```python
from build123d import *

# Parameters (mm, degrees)
F0_W      = 38.1
F0_H      = 38.1
F1_DEPTH  = 38.1
F6_DEPTH  = 38.1
F8_DEPTH  = 38.1
F9_W      = 25.4
F9_H      = 7.62
F10_DEPTH = 38.1


with BuildPart() as f1:
    # F0 (on Front) → F1 (new body)
    with BuildSketch(Plane.XZ):
        with Locations((-19.05, 19.05)):
            Rectangle(F0_W, F0_H)
    extrude(amount=F1_DEPTH)

    # F5 (on offset) → F6 (cut)
    with BuildSketch(Plane.YZ.offset(-38.1)):
        Polygon((-11.43, 13.500985), (-6.35, 38.1), (-31.75, 38.1), (-26.67, 13.624078), (-21.59, 28.575), (-16.51, 28.575), align=None)
        Polygon((-25.4, 0), (-12.7, 0), (-19.05, 15.875), align=None)
        Polygon((-6.35, 0), (0, 0), (0, 38.1), align=None)
        Polygon((-31.75, 0), (-38.1, 38.1), (-38.1, 0), align=None)
    extrude(amount=F6_DEPTH, mode=Mode.SUBTRACT)

    # F7 (on offset) → F8 (cut)
    with BuildSketch(Plane.XZ.offset(38.1)):
        Polygon((-31.75, 0), (-6.35, 0), (-11.43, 19.455044), (-16.51, 9.525), (-21.59, 9.525), (-26.67, 19.085767), align=None)
        Polygon((-6.35, 38.1), (0, 0), (0, 38.1), align=None)
        Polygon((-19.05, 22.225), (-12.7, 38.1), (-25.4, 38.1), align=None)
        Polygon((-38.1, 38.1), (-38.1, 0), (-31.75, 38.1), align=None)
    extrude(amount=-F8_DEPTH, mode=Mode.SUBTRACT)

    # F9 (on offset) → F10 (cut)
    with BuildSketch(Plane.XY.offset(38.1)):
        with Locations((-12.7, -11.43)):
            Rectangle(F9_W, F9_H)
        with Locations((-25.4, -26.67)):
            Rectangle(F9_W, F9_H)
    extrude(amount=-F10_DEPTH, mode=Mode.SUBTRACT)


solid = f1.part
```
For this review, take the finished solid that the model builds, in its own axes (mm). A direction names the side the tool comes from. Round coordinates to 2 decimals unless told otherwise and drop trailing zeros. Write each loop counter-clockwise with the first axis right and the second up, starting at its lowest first coordinate (ties: lowest second). Pieces come first, ordered by that corner, then holes. Notation, with made-up numbers: (16, 5) - (55, 5) arc R6 cw to (55, 9) - close; hole circle Ø10 at (43, 80.25). An arc over 180 degrees is marked (long way). Answer as CSV lines item,"result". Start each with the question number.
(1) Add section D-D, the plane z = 12. State how many separate pieces and enclosed holes the cut face has, plus the area to 3 significant figures.
(2) For line 1 (Y direction, x = -26.5, z = 23.5); line 2 (Y direction, x = -11.5, z = 21); line 3 (X direction, y = -22.5, z = 10.5), list the stretches that pass through material, from the lowest coordinate up.
(3) Add section A-A, the plane x = -3.5. State the section outline as (y, z) points (3 decimals).
(4) Mouldability with a two-part tool opening along Y and no side actions: class faces 6 (the flat face through (-22.27, -33.5, 30.27)), 7 (the flat face through (-19.32, -34.88, 18.78)), 8 (the flat face through (-26, -30.48, 20)) as +Y half, -Y half, draft (parallel to the pull), parting line (faces both ways), or undercut.
(5) Add section B-B, the plane z = 30.5. State the section outline as (x, y) points, plus the area to 3 significant figures.
(6) Add section C-C, the plane y = -9.5. State the section outline as (x, z) points.
(7) For pin 1 (2 mm diameter, centred on x = -32, z = 10, fed in from -Y); pin 2 (2.5 mm diameter, centred on x = -13, y = -18.5, fed in from +Z) (3 decimals); pin 3 (8 mm diameter, centred on x = -28.5, y = -34, fed in from -Z); pin 4 (2 mm diameter, centred on y = -23.5, z = 19.5, fed in from -X), all flat-tipped, find the tip position at first contact; note any pin that passes through.
(8) Machinability: for faces 1 (the flat face through (-4, -5, 24)), 2 (the flat face through (-13.934, -5.897, 14.56)), 3 (the flat face through (-27.93, -31.124, 35.083)), 4 (the flat face through (-15.9, -33.5, 30.1)), 5 (the flat face through (-19.195, -18.044, 13.361)), which of the approach directions +Z, -Z, +X, -X, +Y, -Y give a long, thin tool a straight path to every point of the face, cutting with its end or side? Answer none if there is none.
From the geometry:
1,separate pieces,"10"
1,enclosed holes,"0"
1,area,"365 mm²"
2,line 1,"y = -35.67 to -30.48, -22.86 to -14.8, -9.37 to -2.43"
2,line 2,"y = -35.25 to -28.2, -24.16 to -15.24, -7.62 to -2.85"
2,line 3,"x = -36.35 to -28.96, -22.11 to -16.01, -9.09 to -1.75"
3,outline,"(-35.25, 21) - (-31.75, 0) - (-25.4, 0) - (-19.05, 15.875) - (-15.24, 6.35) - (-15.24, 21) - (-24.164, 21) - (-26.67, 13.624) - (-28.201, 21) - close; (-7.62, 0) - (-6.35, 0) - (-2.85, 21) - (-7.62, 21) - close"
4,face 6,"draft"
4,face 7,"-Y half"
4,face 8,"undercut"
5,outline,"(-33.02, -36.83) - (-22.36, -36.83) - (-22.36, -30.48) - (-33.02, -30.48) - close; (-33.02, -7.92) - (-25.4, -7.92) - (-25.4, -7.62) - (-22.36, -7.62) - (-22.36, -1.27) - (-33.02, -1.27) - close; (-15.74, -36.83) - (-5.08, -36.83) - (-5.08, -30.17) - (-12.7, -30.17) - (-12.7, -30.48) - (-15.74, -30.48) - close; (-15.74, -7.62) - (-5.08, -7.62) - (-5.08, -1.27) - (-15.74, -1.27) - close"
5,area,"275 mm²"
6,outline,"(-38.1, 0) - (-31.75, 0) - (-26.67, 19.09) - (-25.4, 16.7) - (-25.4, 22.85) - (-34.29, 22.85) - close"
7,pin 1,"stops at y = -33.58"
7,pin 2,"stops at z = 28.575"
7,pin 3,"stops at z = 0"
7,pin 4,"stops at x = -34.98"
8,face 1,"+Z, +X, +Y, -Y"
8,face 2,"-Z, +Y, -Y"
8,face 3,"+Z, +X, -X"
8,face 4,"+Z, +Y, -Y"
8,face 5,"-Z, +X, -X"
